Input: part model. Units: mm. Frame: model coordinates. A direction names the side the tool comes from. Give positions to 0.01 mm unless a question says otherwise; leave off trailing zeros. Order: outer loops, then holes, each group sorted by start corner. A loop starts at its lowest first (then second) coordinate and runs counter-clockwise, first axis right, second up. Notation, with made-up numbers: M 48.25,0 L 59.25,0 A22 ccw 59.25,17 Z; hole C 15.25,8.25 d6. An arc over 180 degrees is marked long. Use a Markdown table: item, result.
from build123d import *

# Parameters (mm, degrees)
SKETCH1_R                                            = 87.5
BOSS_EXTRUDE1_DEPTH                                  = 5
SKETCH2_R                                            = 84.325
CUT_EXTRUDE1_DEPTH                                   = 1.825
SKETCH3_R                                            = 6
SKETCH3_W                                            = 8.5
SKETCH3_H                                            = 8.5
CUT_EXTRUDE2_DEPTH                                   = 124.784411882
SKETCH4_R                                            = 2.5
BOSS_EXTRUDE2_DEPTH                                  = 4.325
SKETCH4_2_R                                          = 2.5
BOSS_EXTRUDE3_DEPTH                                  = 9.625
CSK_FOR_M2_5_CROSS_COUNTERSUNK_HEAD_SCRE_D           = 2.9
CSK_FOR_M2_5_CROSS_COUNTERSUNK_HEAD_SCRE_CSINK_D     = 5
CSK_FOR_M2_5_CROSS_COUNTERSUNK_HEAD_SCRE_CSINK_ANGLE = 92
CSK_FOR_M2_CROSS_COUNTERSUNK_HEAD_SCREW1_D           = 2.4
CSK_FOR_M2_CROSS_COUNTERSUNK_HEAD_SCREW1_CSINK_D     = 4
CSK_FOR_M2_CROSS_COUNTERSUNK_HEAD_SCREW1_CSINK_ANGLE = 92


with BuildPart() as part:
    # Sketch1 → Boss-Extrude1 (new body)
    with BuildSketch(Plane(origin=(0, 0, 0), x_dir=(1, 0, 0), z_dir=(0, 1, 0))):
        with Locations(Location((0, 0, 0), (0, 0, 270))):
            Circle(SKETCH1_R)
    extrude(amount=BOSS_EXTRUDE1_DEPTH)

    # Sketch2 → Cut-Extrude1 (cut)
    with BuildSketch(Plane(origin=(0, 5, 0), x_dir=(1, 0, 0), z_dir=(0, 1, 0))):
        with Locations(Location((0, 0, 0), (0, 0, 270))):
            Circle(SKETCH2_R)
    extrude(amount=-CUT_EXTRUDE1_DEPTH, mode=Mode.SUBTRACT)

    # Sketch3 → Cut-Extrude2 (cut, through all)
    with BuildSketch(Plane(origin=(0, 3.175, 0), x_dir=(1, 0, 0), z_dir=(0, 1, 0))):
        with Locations(Location((23, -16.5546, 0), (0, 0, 270))):
            Circle(SKETCH3_R)
        with Locations((0, -16.8926)):
            Rectangle(SKETCH3_W, SKETCH3_H)
    extrude(amount=-CUT_EXTRUDE2_DEPTH, mode=Mode.SUBTRACT)

    # Sketch4 → Boss-Extrude2 (add)
    with BuildSketch(Plane(origin=(0, 3.175, 0), x_dir=(1, 0, 0), z_dir=(0, 1, 0))):
        with Locations(Location((10.5, -4.4926, 0), (0, 0, 270))):
            Circle(SKETCH4_R)
        with Locations(Location((10.5, -16.9926, 0), (0, 0, 270))):
            Circle(SKETCH4_R)
        with Locations(Location((-10.5, -16.9926, 0), (0, 0, 270))):
            Circle(SKETCH4_R)
        with Locations(Location((-10.5, -4.4926, 0), (0, 0, 270))):
            Circle(SKETCH4_R)
    extrude(amount=BOSS_EXTRUDE2_DEPTH)

    # Sketch4_2 → Boss-Extrude3 (add)
    with BuildSketch(Plane(origin=(0, 3.175, 0), x_dir=(1, 0, 0), z_dir=(0, 1, 0))):
        with Locations(Location((27.5, 3.3254, 0), (0, 0, 270))):
            Circle(SKETCH4_2_R)
        with Locations(Location((27.5, -45.6746, 0), (0, 0, 270))):
            Circle(SKETCH4_2_R)
        with Locations(Location((18.5, -45.6746, 0), (0, 0, 270))):
            Circle(SKETCH4_2_R)
        with Locations(Location((18.5, 3.3254, 0), (0, 0, 270))):
            Circle(SKETCH4_2_R)
    extrude(amount=BOSS_EXTRUDE3_DEPTH)

    # CSK for M2.5 Cross Countersunk Head Scre (through all)
    with Locations(Plane(origin=(0, 0, 0), x_dir=(-1, 0, 0), z_dir=(0, -1, 0))):
        with Locations((-27.5, 3.3254), (-18.5, 3.3254), (-27.5, -45.6746), (-18.5, -45.6746)):
            CounterSinkHole(CSK_FOR_M2_5_CROSS_COUNTERSUNK_HEAD_SCRE_D / 2, CSK_FOR_M2_5_CROSS_COUNTERSUNK_HEAD_SCRE_CSINK_D / 2, counter_sink_angle=CSK_FOR_M2_5_CROSS_COUNTERSUNK_HEAD_SCRE_CSINK_ANGLE)

    # CSK for M2 Cross Countersunk Head Screw1 (through all)
    with Locations(Plane(origin=(0, 0, 0), x_dir=(-1, 0, 0), z_dir=(0, -1, 0))):
        with Locations((10.5, -4.4926), (-10.5, -4.4926), (-10.5, -16.9926), (10.5, -16.9926)):
            CounterSinkHole(CSK_FOR_M2_CROSS_COUNTERSUNK_HEAD_SCREW1_D / 2, CSK_FOR_M2_CROSS_COUNTERSUNK_HEAD_SCREW1_CSINK_D / 2, counter_sink_angle=CSK_FOR_M2_CROSS_COUNTERSUNK_HEAD_SCREW1_CSINK_ANGLE)


solid = part.part
1) Mould query, pull axis X, two halves, no side actions, for faces 3 (the face through (1, 3.175, -1)), 4 (the face through (-12.718, 5.307, 18.146)), 5 (the face through (17, 12.8, -2)). Classes: released by +X, released by -X, zero draft, split by the parting line, or undercut.
Response values:
| item | result |
|---|---|
| face 3 | undercut |
| face 4 | undercut |
| face 5 | zero draft |
2) First-contact query: pin 1 Ø1 at (y, z) = (2, 15.5) entering from +X; pin 2 Ø10 at (x, z) = (-45.5, -45) entering from +Y (3 decimals); pin 3 Ø4 at (x, z) = (-9.5, 17) entering from +Y. Flat tips, straight axial feed; report the tip coordinate or a pass-through.
Response values:
| item | result |
|---|---|
| pin 1 | stops at x = 86.2 |
| pin 2 | stops at y = 3.175 |
| pin 3 | stops at y = 7.5 |
3) Material intervals for line 1 (Z direction, x = 1.5, y = 2.75); line 2 (X direction, y = 2.25, z = 19.5); line 3 (X direction, y = 3.6, z = 0) (3 decimals), sorted ascending. Write a range as from..to.
Response values:
| item | result |
|---|---|
| line 1 | z = -87.49..12.64, 21.14..87.49 |
| line 2 | x = -85.3..-4.25, 4.25..17.77, 28.23..85.3 |
| line 3 | x = -87.5..-84.325, 84.325..87.5 |
4) Cut plane A-A on y = 10. Return loops of the section in (x, z), and give its area (3 significant figures).
Response values:
| item | result |
|---|---|
| outline | C 18.5,-3.33 d5; C 18.5,45.67 d5; C 27.5,-3.33 d5; C 27.5,45.67 d5; hole C 18.5,-3.33 d2.9; hole C 18.5,45.67 d2.9; hole C 27.5,-3.33 d2.9; hole C 27.5,45.67 d2.9 |
| area | 52.1 mm² |
5) Cut plane C-C on z = -68.5. Return loops of the section in (x, y) (3 decimals).
Response values:
| item | result |
|---|---|
| outline | M -54.443,0 L 54.443,0 L 54.443,5 L 49.178,5 L 49.178,3.175 L -49.178,3.175 L -49.178,5 L -54.443,5 Z |
6) Cut plane B-B on x = 23. Return loops of the section in (y, z) (3 decimals).
Response values:
| item | result |
|---|---|
| outline | M 0,-84.423 L 5,-84.423 L 5,-81.128 L 3.175,-81.128 L 3.175,10.555 L 0,10.555 Z; M 0,22.555 L 3.175,22.555 L 3.175,81.128 L 5,81.128 L 5,84.423 L 0,84.423 Z |
7) Cut plane D-D on x = -29.5. Return loops of the section in (y, z) (3 decimals), and give its area (3 significant figures).
Response values:
| item | result |
|---|---|
| outline | M 0,-82.377 L 5,-82.377 L 5,-78.997 L 3.175,-78.997 L 3.175,78.997 L 5,78.997 L 5,82.377 L 0,82.377 Z |
| area | 535 mm² |
8) Reachability of faces 1 (the face through (29.98, 7.92, -3.65)), 2 (the face through (-12, 7.5, 4)) from +Z, -Z, +X, -X, +Y, -Y: full face, straight path, thin tool, end or side. Return the list, or none.
Response values:
| item | result |
|---|---|
| face 1 | +Y |
| face 2 | +Z, -Z, +X, -X, +Y |
